Could you check a few things on this model? Use its own coordinates, in mm. A direction names the side the tool comes from. Round coordinates to 2 decimals unless told otherwise and drop trailing zeros. Write each loop counter-clockwise with the first axis right and the second up, starting at its lowest first coordinate (ties: lowest second). Pieces come first, ordered by that corner, then holes. Notation, with made-up numbers: (18, 71.25) -> (44, 71.25) arc R20 cw to (44, 94.25) -> close; hole circle Ø2 at (53.5, 11.5). An arc over 180 degrees is marked (long way). Answer in a Markdown table with one row per item.
from build123d import *

# Parameters (mm, degrees)
EXTRUDE_1_DEPTH     = 22
SKETCH_5_R          = 1.3
CUT_EXTRUDE_2_DEPTH = 19
FILLET_1_R          = 3
SKETCH_6_R          = 1.5
CUT_EXTRUDE_3_DEPTH = 30
SKETCH_7_R          = 1.6
SKETCH_7_R_2        = 0.8
CUT_EXTRUDE_4_DEPTH = 27
FILLET_2_R          = 3


with BuildPart() as part:
    # 草图1 → 凸台-拉伸1 (new body)
    with BuildSketch(Plane.XY):
        Polygon((0, 12.829776804), (0, 10.829776804), (10, 10.829776804), (10, 5.129776804), (12, 5.129776804), (17.5, 4.129776804), (22.5, 4.129776804), (22.5, 5.129776804), (17.5, 5.129776804), (12, 12.829776804), align=None)
    extrude_1 = extrude(amount=EXTRUDE_1_DEPTH)

    # 镜向1: 凸台-拉伸1 across plane
    add(extrude_1.mirror(Plane(origin=(0, 0, 22), x_dir=(0, 0, 1), z_dir=(1, 0, 0))))

    # 草图5 → 切除-拉伸2 (cut)
    with BuildSketch(Plane(origin=(0, 0, 0), x_dir=(1, 0, 0), z_dir=(0, 1, 0))):
        with Locations((-20, -3)):
            Circle(SKETCH_5_R)
        with Locations((-20, -19)):
            Circle(SKETCH_5_R)
        with Locations(Location((20, -3, 0), (0, 0, 270))):
            Circle(SKETCH_5_R)
        with Locations(Location((20, -19, 0), (0, 0, 270))):
            Circle(SKETCH_5_R)
    extrude(amount=CUT_EXTRUDE_2_DEPTH, mode=Mode.SUBTRACT)

    # 圆角1
    fillet_1_edges = [part.edges().sort_by_distance(p)[0] for p in [
        (22.5, 4.629776804, 0),
        (22.5, 4.629776804, 22),
        (-22.5, 4.629776804, 22),
        (-22.5, 4.629776804, 0),
    ]]
    fillet(fillet_1_edges, radius=FILLET_1_R)

    # 草图6 → 切除-拉伸3 (cut)
    with BuildSketch(Plane(origin=(0, 0, 0), x_dir=(1, 0, 0), z_dir=(0, 1, 0))):
        with Locations(Location((-3, -8, 0), (0, 0, 270))):
            Circle(SKETCH_6_R)
        with Locations(Location((-7.5, -8, 0), (0, 0, 270))):
            Circle(SKETCH_6_R)
        with Locations(Location((-7.5, -3.5, 0), (0, 0, 270))):
            Circle(SKETCH_6_R)
        with Locations(Location((-3, -3.5, 0), (0, 0, 270))):
            Circle(SKETCH_6_R)
        with Locations(Location((-3, -14, 0), (0, 0, 270))):
            Circle(SKETCH_6_R)
        with Locations(Location((-7.5, -14, 0), (0, 0, 270))):
            Circle(SKETCH_6_R)
        with Locations(Location((-3, -18.5, 0), (0, 0, 270))):
            Circle(SKETCH_6_R)
        with Locations(Location((-7.5, -18.5, 0), (0, 0, 270))):
            Circle(SKETCH_6_R)
        with Locations(Location((3, -18.5, 0), (0, 0, 270))):
            Circle(SKETCH_6_R)
        with Locations(Location((7.5, -18.5, 0), (0, 0, 270))):
            Circle(SKETCH_6_R)
        with Locations(Location((3, -14, 0), (0, 0, 270))):
            Circle(SKETCH_6_R)
        with Locations(Location((7.5, -14, 0), (0, 0, 270))):
            Circle(SKETCH_6_R)
        with Locations(Location((3, -8, 0), (0, 0, 270))):
            Circle(SKETCH_6_R)
        with Locations(Location((7.5, -8, 0), (0, 0, 270))):
            Circle(SKETCH_6_R)
        with Locations(Location((3, -3.5, 0), (0, 0, 270))):
            Circle(SKETCH_6_R)
        with Locations(Location((7.5, -3.5, 0), (0, 0, 270))):
            Circle(SKETCH_6_R)
    extrude(amount=CUT_EXTRUDE_3_DEPTH, mode=Mode.SUBTRACT)

    # 草图7 → 切除-拉伸4 (cut)
    with BuildSketch(Plane.XY):
        with Locations((12.426108542, 7.644425741)):
            Circle(SKETCH_7_R)
        with Locations((15.018691649, 5.985664037)):
            Circle(SKETCH_7_R_2)
        with Locations((11.76260386, 10.593335436)):
            Circle(SKETCH_7_R_2)
        with Locations(Location((-11.76260386, 10.593335436, 0), (0, 0, 180))):
            Circle(SKETCH_7_R_2)
        with Locations(Location((-12.426108542, 7.644425741, 0), (0, 0, 180))):
            Circle(SKETCH_7_R)
        with Locations(Location((-15.018691649, 5.985664037, 0), (0, 0, 180))):
            Circle(SKETCH_7_R_2)
    extrude(amount=CUT_EXTRUDE_4_DEPTH, mode=Mode.SUBTRACT)

    # 圆角2
    fillet_2_edges = [part.edges().sort_by_distance(p)[0] for p in [
        (12, 12.829776804, 11),
        (-12, 12.829776804, 11),
    ]]
    fillet(fillet_2_edges, radius=FILLET_2_R)


solid = part.part
1) For pin 1 (3.5 mm diameter, centred on x = -3, z = 8, fed in from -Y); pin 2 (3.5 mm diameter, centred on x = 20, z = 19, fed in from +Y); pin 3 (2 mm diameter, centred on x = 16, z = 11.5, fed in from +Y), each with a flat end and sliding along its axis, tell me the tip position at first contact or that it passes through.
Findings:
| item | result |
|---|---|
| pin 1 | stops at y = 10.83 |
| pin 2 | stops at y = 5.13 |
| pin 3 | stops at y = 8.63 |
2) For faces 5 (the face through (-20, 5.13, 11)), 6 (the face through (11, 5.13, 11)), 7 (the face through (-12.193, 9.919, 10.846)), which set-ups out of +Z, -Z, +X, -X, +Y, -Y let a thin tool reach every point of the face, with its end or its side?
Findings:
| item | result |
|---|---|
| face 5 | +Z, -Z, -X, +Y |
| face 6 | +Z, -Z, -Y |
| face 7 | +Z, -Z |
3) Please list where these lines run through material, in increasing order: line 1 (Z direction, x = -7.5, y = 11.45); line 2 (X direction, y = 6, z = 10); line 3 (X direction, y = 5.5, z = 7.5).
Findings:
| item | result |
|---|---|
| line 1 | z = 0 to 2, 5 to 6.5, 9.5 to 12.5, 15.5 to 17, 20 to 22 |
| line 2 | x = -16.88 to -15.82, -14.22 to -10, 10 to 14.22, 15.82 to 16.88 |
| line 3 | x = -17.24 to -15.65, -14.38 to -10, 10 to 14.38, 15.65 to 17.24 |
4) Thinking about a two-plate mould opening in X: for faces 1 (the face through (-15.23, 8.31, 10.85)), 2 (the face through (0, 11, 22)), 3 (the face through (-14.712, 4.637, 10.846)), 4 (the face through (15.23, 8.31, 10.85)), which applies, +X half, -X half, draft (parallel to the pull), parting line (faces both ways), or undercut?
Findings:
| item | result |
|---|---|
| face 1 | -X half |
| face 2 | draft |
| face 3 | undercut |
| face 4 | +X half |
5) Imagine slicing it at B-B, the plane x = 20. Please give me the cut outline in (y, z), plus the area to 3 significant figures.
Findings:
| item | result |
|---|---|
| outline | (4.13, 0.04) -> (5.13, 0.04) -> (5.13, 1.7) -> (4.13, 1.7) -> close; (4.13, 4.3) -> (5.13, 4.3) -> (5.13, 17.7) -> (4.13, 17.7) -> close; (4.13, 20.3) -> (5.13, 20.3) -> (5.13, 21.96) -> (4.13, 21.96) -> close |
| area | 16.7 mm^2 |
6) Imagine slicing it at A-A, the plane x = 3. Please give me the cut outline in (y, z).
Findings:
| item | result |
|---|---|
| outline | (10.83, 0) -> (12.83, 0) -> (12.83, 2) -> (10.83, 2) -> close; (10.83, 5) -> (12.83, 5) -> (12.83, 6.5) -> (10.83, 6.5) -> close; (10.83, 9.5) -> (12.83, 9.5) -> (12.83, 12.5) -> (10.83, 12.5) -> close; (10.83, 15.5) -> (12.83, 15.5) -> (12.83, 17) -> (10.83, 17) -> close; (10.83, 20) -> (12.83, 20) -> (12.83, 22) -> (10.83, 22) -> close |
7) Imagine slicing it at D-D, the plane z = 10.5. Please give me the cut outline in (x, y), plus the area to 3 significant figures.
Findings:
| item | result |
|---|---|
| outline | (-22.5, 4.13) -> (-17.5, 4.13) -> (-12, 5.13) -> (-10, 5.13) -> (-10, 10.83) -> (10, 10.83) -> (10, 5.13) -> (12, 5.13) -> (17.5, 4.13) -> (22.5, 4.13) -> (22.5, 5.13) -> (17.5, 5.13) -> (12.9, 11.57) arc R3 ccw to (10.46, 12.83) -> (-10.46, 12.83) arc R3 ccw to (-12.9, 11.57) -> (-17.5, 5.13) -> (-22.5, 5.13) -> close; hole circle Ø1.6 at (-15.02, 5.99); hole circle Ø3.2 at (-12.43, 7.64); hole circle Ø1.6 at (-11.76, 10.59); hole circle Ø3.2 at (12.43, 7.64); hole circle Ø1.6 at (11.76, 10.59); hole circle Ø1.6 at (15.02, 5.99) |
| area | 104 mm^2 |
8) Imagine slicing it at C-C, the plane z = 13.75. Count the separate pieces of the cut face and the enclosed holes in it, plus the area to 4 significant figures.
Findings:
| item | result |
|---|---|
| separate pieces | 5 |
| enclosed holes | 6 |
| area | 80.15 mm^2 |
